Check sheet for the modelled part. Datum: model origin and axes. Units: mm. A direction names the side the tool comes from. Coordinates: 2 decimals unless noted, no trailing zeros. Loops run counter-clockwise (first coordinate to the right, second up) from the corner with the lowest first, then second, coordinate; pieces in that order, holes last. Notation, with made-up numbers: M 82,-7.75 L 106,-7.75 A28 ccw 106,15.25 Z; hole C 10.25,5 d7. An arc over 180 degrees is marked long. Return JSON: item names as keys, results as strings.
from build123d import *

# Parameters (mm, degrees)
SKETCH_R      = 7.5
SKETCH_R_2    = 6.15
PAD_DEPTH     = 2
SKETCH001_R   = 6.65
SKETCH001_R_2 = 6.15
PAD001_DEPTH  = 36
SKETCH002_W   = 42.259399
SKETCH002_H   = 12
POCKET_DEPTH  = 17.501


with BuildPart() as part:
    # Sketch → Pad (new body)
    with BuildSketch(Plane.XY):
        Circle(SKETCH_R)
        Circle(SKETCH_R_2, mode=Mode.SUBTRACT)
    extrude(amount=PAD_DEPTH)

    # Sketch001 (on Face4 of Pad) → Pad001 (join)
    with BuildSketch(Plane.XY.offset(2)):
        Circle(SKETCH001_R)
        Circle(SKETCH001_R_2, mode=Mode.SUBTRACT)
    extrude(amount=PAD001_DEPTH)

    # Sketch002 (on DatumPlane) → Pocket (cut, through all)
    with BuildSketch(Plane(origin=(10, 0, 0), x_dir=(0, 0, -1), z_dir=(1, 0, 0))):
        with Locations((-23.129699, 0)):
            Rectangle(SKETCH002_W, SKETCH002_H)
    extrude(amount=-POCKET_DEPTH, mode=Mode.SUBTRACT)


solid = part.part
1) Section check C-C on z = 22. Record the cut outline in (x, y).
Answers:
{"outline": "M -2.87,-6 A6.65 ccw 2.87,-6 L 1.35,-6 A6.15 cw -1.35,-6 Z; M -2.87,6 L -1.35,6 A6.15 cw 1.35,6 L 2.87,6 A6.65 ccw Z"}
2) Section check A-A on x = 0. Record the cut outline in (y, z), then the cut area to 3 significant figures.
Answers:
{"outline": "M -7.5,0 L -6.15,0 L -6.15,38 L -6.65,38 L -6.65,2 L -7.5,2 Z; M 6.15,0 L 7.5,0 L 7.5,2 L 6.65,2 L 6.65,38 L 6.15,38 Z", "area": "41.4 mm²"}
3) Draft check along X on faces 4 (the face through (2, 6, 20)), 5 (the face through (-0.98, 6.07, 14.69)), 6 (the face through (-0.04, -6.65, 19.75)). Enter one of: +X half, -X half, draft (parallel to the pull), parting line (faces both ways), or undercut.
Answers:
{"face 4": "draft", "face 5": "undercut", "face 6": "parting line"}
4) Go/stop test with flat-tipped pins: pin 1 Ø7 at (x, y) = (-3, -1) entering from +Z; pin 2 Ø2.5 at (x, z) = (3, 21.5) entering from -Y; pin 3 Ø1 at (x, z) = (-3.5, 21.5) entering from -Y; pin 4 Ø4 at (x, z) = (4.5, 27.5) entering from -Y. Record where each tip stops, or that it passes through.
Answers:
{"pin 1": "z = 2", "pin 2": "y = -6.42", "pin 3": "through", "pin 4": "y = -6.16"}
5) Set-up check for faces 1 (the face through (2, -6, 20)), 2 (the face through (0, -7, 2)), 3 (the face through (0.04, 6.65, 19.75)): record each of +Z, -Z, +X, -X, +Y, -Y from which the full face is reachable in a straight line by a thin tool's end or side.
Answers:
{"face 1": "+Z, +X, -X", "face 2": "+Z, -Y", "face 3": "+Z, +Y"}
6) Section check D-D on x = 1.75. Record the cut outline in (y, z).
Answers:
{"outline": "M -7.29,0 L -5.9,0 L -5.9,2 L -6,2 L -6,38 L -6.42,38 L -6.42,2 L -7.29,2 Z; M 5.9,0 L 7.29,0 L 7.29,2 L 6.42,2 L 6.42,38 L 6,38 L 6,2 L 5.9,2 Z"}
7) Section check B-B on y = 0. Record the cut outline in (x, z), then the cut area to 3 significant figures.
Answers:
{"outline": "M -7.5,0 L -6.15,0 L -6.15,2 L -7.5,2 Z; M 6.15,0 L 7.5,0 L 7.5,2 L 6.15,2 Z", "area": "5.40 mm²"}
8) Scan lines: line 1 along Y through (x, z) = (1.5, 13.5); line 2 along Z through (x, y) = (5.5, -4.5); line 3 along Y through (x, z) = (2, 33). Record each from-to range of solid material in increasing order. Write a range as [from, to].
Answers:
{"line 1": "[-6.48, -6], [6, 6.48]", "line 2": "[0, 2]", "line 3": "[-6.34, -6], [6, 6.34]"}
